Answer from the drawing. Dimensions are ordinates in mm from the lowest x, y and z of the part. Round coordinates to 2 decimals unless told otherwise and drop trailing zeros. Write each loop counter-clockwise with the first axis right and the second up, starting at its lowest first coordinate (ties: lowest second). Pieces come first, ordered by that corner, then holes.
1. Find section B-B (x = 32.5). Write down the section's boundary in (y, z), and give its area (3 significant figures).
2. Flat-ended cylindrical pins translate along their axes: pin 1 Ø1 at (y, z) = (13.5, 1.5) entering from -X; pin 2 Ø3.5 at (x, y) = (81, 21.5) entering from +Z. Find the tip coordinate at first contact, or state that the pin passes through.
3. Find section A-A (x = 107.5). Write down the section's boundary in (y, z).
4. Straight lines are drawn through the part: probe 1 along X at (y, z) = (20, 5.25); probe 2 along X at (y, z) = (20, 9.1); probe 3 along Y at (x, z) = (32.5, 8.45). For each, find the intervals that lie inside material, in ascending order.
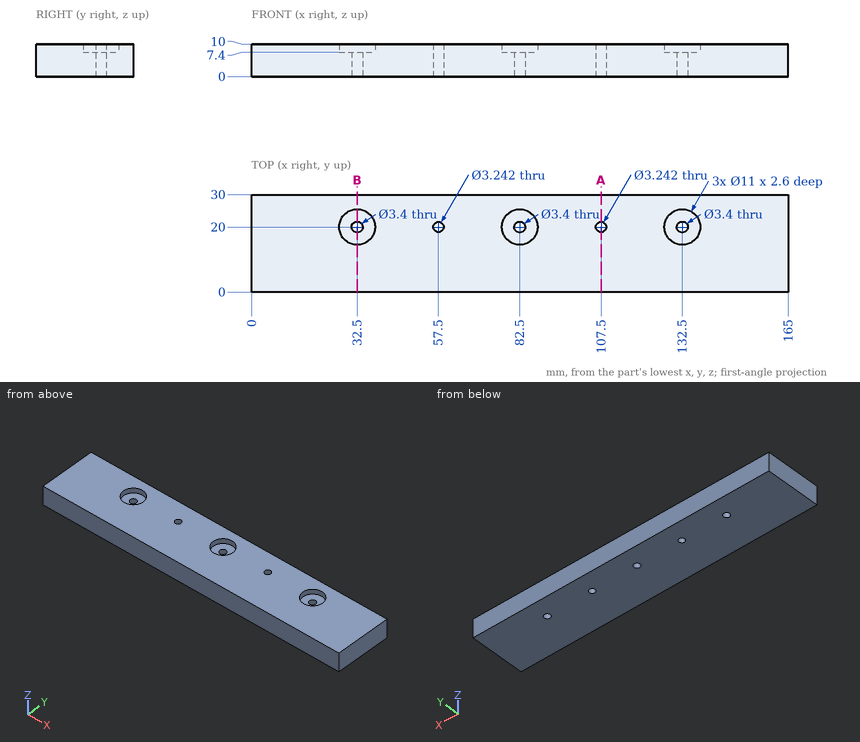
Worked answers:
1. outline: (0, 0) - (18.3, 0) - (18.3, 7.4) - (14.5, 7.4) - (14.5, 10) - (0, 10) - close; (21.7, 0) - (30, 0) - (30, 10) - (25.5, 10) - (25.5, 7.4) - (21.7, 7.4) - close
1. area: 246 mm2
2. pin 1: stops at x = 0
2. pin 2: stops at z = 7.4
3. outline: (0, 0) - (18.38, 0) - (18.38, 10) - (0, 10) - close; (21.62, 0) - (30, 0) - (30, 10) - (21.62, 10) - close
4. probe 1: x = 0 to 30.8, 34.2 to 55.88, 59.12 to 80.8, 84.2 to 105.88, 109.12 to 130.8, 134.2 to 165
4. probe 2: x = 0 to 27, 38 to 55.88, 59.12 to 77, 88 to 105.88, 109.12 to 127, 138 to 165
4. probe 3: y = 0 to 14.5, 25.5 to 30
